Check sheet for the modelled part. Datum: model origin and axes. Units: mm. A direction names the side the tool comes from. Give positions to 0.01 mm unless a question says otherwise; leave off trailing zeros. Order: outer loops, then holes, each group sorted by start corner. A loop starts at its lowest first (then second) coordinate and runs counter-clockwise, first axis right, second up. Notation, with made-up numbers: (-18, -16) -> (30, -16) arc R26 ccw to (30, 1) -> close; hole circle Ø5 at (29.5, 34). An arc over 180 degrees is marked (long way). Write each question's results on one line, items separated by ' | '.
from build123d import *

# Parameters (mm, degrees)
SKETCH1_R           = 3
SKETCH1_W           = 2
SKETCH1_H           = 1.17
BOSS_EXTRUDE1_DEPTH = 30
SKETCH2_R           = 6.166150273
SKETCH2_R_2         = 1.95
CUT_EXTRUDE1_DEPTH  = 22
CUT_EXTRUDE2_DEPTH  = 7
CUT_EXTRUDE3_DEPTH  = 100
SKETCH5_R           = 1.95
CUT_EXTRUDE4_DEPTH  = 2


with BuildPart() as part:
    # Sketch1 → Boss-Extrude1 (new body)
    with BuildSketch(Plane(origin=(0, 0, 0), x_dir=(1, 0, 0), z_dir=(0, 1, 0))):
        Circle(SKETCH1_R)
        with Locations((0, 3.413427125)):
            Rectangle(SKETCH1_W, SKETCH1_H)
    extrude(amount=BOSS_EXTRUDE1_DEPTH)

    # Sketch2 → Cut-Extrude1 (cut)
    with BuildSketch(Plane(origin=(0, 30, 0), x_dir=(1, 0, 0), z_dir=(0, 1, 0))):
        Circle(SKETCH2_R)
        Circle(SKETCH2_R_2, mode=Mode.SUBTRACT)
    extrude(amount=-CUT_EXTRUDE1_DEPTH, mode=Mode.SUBTRACT)

    # Sketch3 → Cut-Extrude2 (cut)
    with BuildSketch(Plane(origin=(0, 30, 0), x_dir=(1, 0, 0), z_dir=(0, 1, 0))):
        with BuildLine():
            Line((-0.975, 1.688749537), (-0.975, -1.688749537))
            ThreePointArc((-0.975, -1.688749537), (-1.95, 0), (-0.975, 1.688749537))
        make_face()
        with BuildLine():
            Line((0.975, 1.688749537), (0.975, -1.688749537))
            ThreePointArc((0.975, -1.688749537), (1.95, 0), (0.975, 1.688749537))
        make_face()
    extrude(amount=-CUT_EXTRUDE2_DEPTH, mode=Mode.SUBTRACT)

    # Sketch4 → Cut-Extrude3 (cut)
    with BuildSketch(Plane.XZ):
        with BuildLine():
            Line((-1, -3.998427125), (1, -3.998427125))
            Line((1, -3.998427125), (1, -2.828427125))
            ThreePointArc((1, -2.828427125), (0, 3), (-1, -2.828427125))
            Line((-1, -2.828427125), (-1, -3.998427125))
        make_face()
        with BuildLine():
            Line((-0.9, -2.75680975), (-0.9, -3.898427125))
            Line((-0.9, -3.898427125), (0.9, -3.898427125))
            Line((0.9, -3.898427125), (0.9, -2.75680975))
            ThreePointArc((0.9, -2.75680975), (0, 2.9), (-0.9, -2.75680975))
        make_face(mode=Mode.SUBTRACT)
    extrude(amount=-CUT_EXTRUDE3_DEPTH, mode=Mode.SUBTRACT)

    # Sketch5 → Cut-Extrude4 (cut)
    with BuildSketch(Plane(origin=(0, 8, 0), x_dir=(1, 0, 0), z_dir=(0, 1, 0))):
        with BuildLine():
            Line((-2.76006086, 0.889979801), (-1.708873277, 4.14998829))
            Line((-1.708873277, 4.14998829), (2.174929625, 4.14998829))
            Line((2.174929625, 4.14998829), (2.48458984, 1.495597984))
            ThreePointArc((2.48458984, 1.495597984), (0.332662617, -2.880856745), (-2.76006086, 0.889979801))
        make_face()
        Circle(SKETCH5_R, mode=Mode.SUBTRACT)
    extrude(amount=-CUT_EXTRUDE4_DEPTH, mode=Mode.SUBTRACT)


solid = part.part
1. Access from +Z, -Z, +X, -X, +Y, -Y to the whole of each face (thin tool, end or side, straight path). Record for faces 1 (the flat face through (0.9, 3, -3)), 2 (the flat face through (1.3, 23, 0)), 3 (the cylindrical face through (0.9, 15.5, 1.73)), 4 (the flat face through (-0.975, 27, 0)), 5 (the flat face through (-0.9, 3, -3)).
Verdict:
face 1: -Z, +X, +Y, -Y | face 2: +Z, -Z, +X, +Y | face 3: +Y | face 4: +Z, -Z, -X, +Y | face 5: -Z, -X, +Y, -Y
2. Material ranges on probe 1 along Y at (x, z) = (-2.4, 0.25); probe 2 along X at (y, z) = (27, -1.5) (3 decimals); probe 3 along Z at (x, y) = (-0.9, 10.5), recorded low to high. Write a range as from..to.
Verdict:
probe 1: y = 0..6 | probe 2: x = -0.975..0.975 | probe 3: z = -1.73..1.73
3. Section check B-B on x = 0. Record the cut outline in (y, z).
Verdict:
outline: (0, -3.9) -> (6, -3.9) -> (6, -1.95) -> (30, -1.95) -> (30, 1.95) -> (6, 1.95) -> (6, 2.9) -> (0, 2.9) -> close
4. Section check A-A on z = 0. Record the cut outline in (x, y) (3 decimals).
Verdict:
outline: (-2.9, 0) -> (2.9, 0) -> (2.9, 6) -> (1.95, 6) -> (1.95, 23) -> (0.975, 23) -> (0.975, 30) -> (-0.975, 30) -> (-0.975, 23) -> (-1.95, 23) -> (-1.95, 6) -> (-2.9, 6) -> close
5. Section check D-D on y = 2.75. Record the cut outline in (x, z), then the cut area to 3 significant figures.
Verdict:
outline: (-0.9, -3.9) -> (0.9, -3.9) -> (0.9, -2.76) arc R2.9 ccw (long way) to (-0.9, -2.76) -> close | area: 28.3 mm^2
6. Gauge pin test, flat ends, axial feed: pin 1 Ø1.3 at (y, z) = (2, -3) entering from +X; pin 2 Ø1.3 at (y, z) = (3, -3.5) entering from -X; pin 3 Ø1 at (x, z) = (1, -2.5) entering from -Y; pin 4 Ø0.5 at (x, z) = (-1.5, 0.5) entering from +Y. Record the tip position at first contact, or that the pin passes through.
Verdict:
pin 1: stops at x = 1.7 | pin 2: stops at x = -0.9 | pin 3: stops at y = 0 | pin 4: stops at y = 23
7. Section check C-C on y = 27. Record the cut outline in (x, z) (3 decimals), then the cut area to 3 significant figures.
Verdict:
outline: (-0.975, -1.689) arc R1.95 ccw to (0.975, -1.689) -> (0.975, 1.689) arc R1.95 ccw to (-0.975, 1.689) -> close | area: 7.28 mm^2
